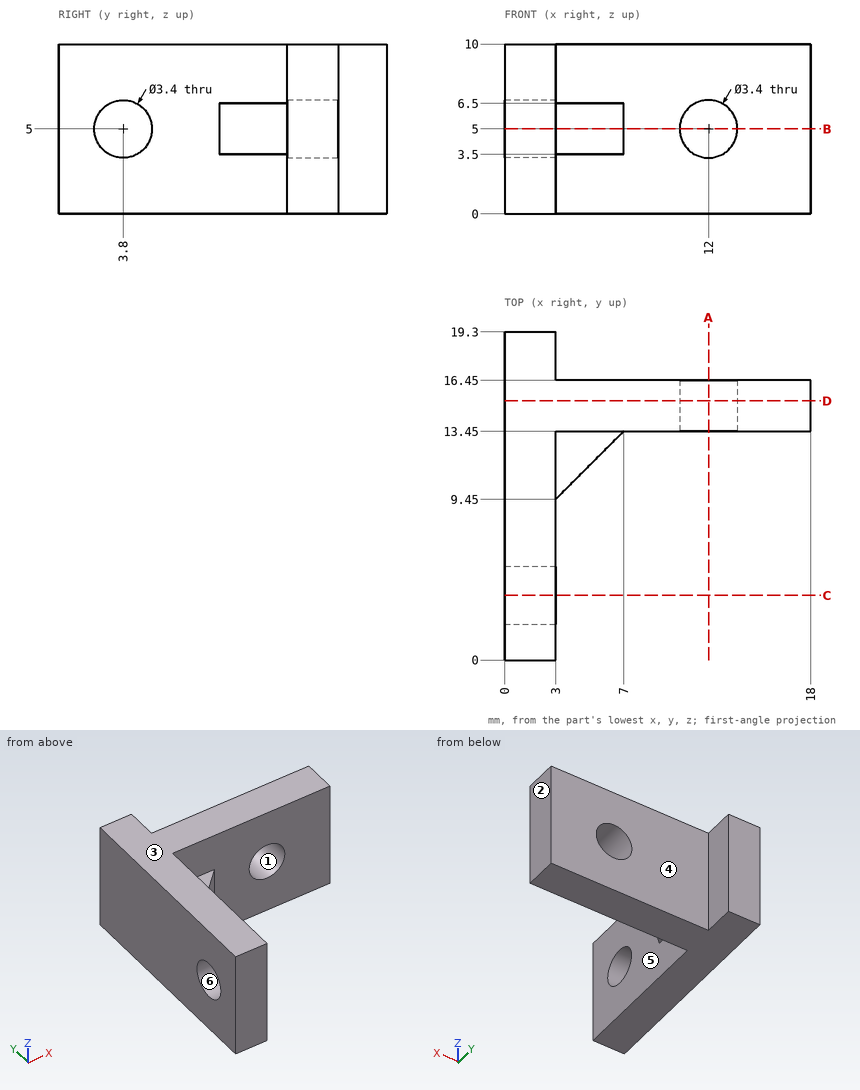
Part print with two shaded views. Sizes in mm from the minimum x, y, z corner. A direction names the side the tool comes from. Coordinates: 2 decimals unless noted, no trailing zeros. Order: outer loops, then holes, each group sorted by start corner. A loop starts at its lowest first (then second) coordinate and runs counter-clockwise, first axis right, second up.
(1) Saw through at A-A, the plane x = 12. Write the cut outline in (y, z).
Solution:
outline: (13.45, 0) - (16.45, 0) - (16.45, 3.3) - (13.45, 3.3) - close; (13.45, 6.7) - (16.45, 6.7) - (16.45, 10) - (13.45, 10) - close
(2) Mould opens along Z. For the marked faces 1, 2 and 3 say: released by +Z, released by -Z, zero draft, split by the parting line, or undercut.
Solution:
face 1: undercut
face 2: zero draft
face 3: released by +Z
(3) Drill centre lines: L1, parallel to X at y = 14.2, z = 5; L2, parallel to Z at x = 1.6, y = 3.8; L3, parallel to X at y = 12, z = 7. Where is each one in solid material? Low to high.
Solution:
L1: x = 0 to 10.3, 13.7 to 18
L2: z = 0 to 3.3, 6.7 to 10
L3: x = 0 to 3
(4) Which spindle directions (+Z, -Z, +X, -X, +Y, -Y) get a long thin tool onto all of the face, cutting with end or side? Do the marked faces 4, 5 and 6. Say none if no direction does.
Solution:
face 4: +Z, -Z, +X, +Y
face 5: +X, -Y
face 6: +X, -X
(5) Saw through at C-C, the plane y = 3.8. Write the cut outline in (x, z), and give its area (3 significant figures).
Solution:
outline: (0, 0) - (3, 0) - (3, 3.3) - (0, 3.3) - close; (0, 6.7) - (3, 6.7) - (3, 10) - (0, 10) - close
area: 19.8 mm2
(6) Saw through at B-B, the plane z = 5. Write the cut outline in (x, y), and give its area (3 significant figures).
Solution:
outline: (0, 0) - (3, 0) - (3, 2.1) - (0, 2.1) - close; (0, 5.5) - (3, 5.5) - (3, 9.45) - (7, 13.45) - (10.3, 13.45) - (10.3, 16.45) - (3, 16.45) - (3, 19.3) - (0, 19.3) - close; (13.7, 13.45) - (18, 13.45) - (18, 16.45) - (13.7, 16.45) - close
area: 90.5 mm2
(7) Pin check, flat tips, straight feed: pin 1 Ø2 at (x, z) = (10.5, 2) entering from +Y; pin 2 Ø5 at (x, z) = (12.5, 4.5) entering from -Y; pin 3 Ø5 at (y, z) = (3.5, 7.5) entering from +X. Stop position of each tip, or through.
Solution:
pin 1: stops at y = 16.45
pin 2: stops at y = 13.45
pin 3: stops at x = 3
(8) Saw through at D-D, the plane y = 15.25. Write the cut outline in (x, z).
Solution:
outline: (0, 0) - (18, 0) - (18, 10) - (0, 10) - close; hole circle Ø3.4 at (12, 5)
